Geometry: final body of the model. Coordinates: model frame, mm. Face numbers are marked on the shaded views. A direction names the side the tool comes from. Give positions to 0.01 mm unless a question says otherwise; leave off trailing zeros. Write each loop counter-clockwise with the first axis right and the second up, starting at its lowest first coordinate (ties: lowest second). Pieces come first, ordered by that corner, then holes.
Q1. Section B-B (x = -79). Return the cut outline in (y, z), plus the area to 3 significant figures.
Q2. Line query: line 1 (Y direction, x = -1.5, z = 42); line 2 (Z direction, x = -93, y = -549.5); line 3 (X direction, y = -310, z = 15). Output: solid intervals per line, ascending.
Q3. Section C-C (y = -154.5). Return the cut outline in (x, z), plus the area to 3 significant figures.
Q4. Section D-D (y = -1123.5). Return the cut outline in (x, z), plus the area to 3 significant figures.
Q5. Section A-A (z = 42). Return the cut outline in (x, y).
Q6. Pin query (flat end, axial travel): pin 1 Ø20.5 at (y, z) = (-846.67, 42) entering from -X; pin 2 Ø3 at (y, z) = (-1386.5, 1.5) entering from -X; pin 3 Ø1.5 at (y, z) = (-871, 23.5) entering from +X; pin 4 Ø16 at (y, z) = (-350, 42) entering from +X. Return the tip coordinate at first contact, or that it passes through.
Q7. Reachability of the marked faces 1 and 2 from +Z, -Z, +X, -X, +Y, -Y: full face, straight path, thin tool, end or side. Return the list, or none.
Autodesk Inventor part; units mm, degrees
ref_plane "YZ Plane" through (0, 0, 0) normal (1, 0, 0) x (0, 1, 0)
ref_plane "XZ Plane" through (0, 0, 0) normal (0, 1, 0) x (-1, 0, 0)
ref_plane "XY Plane" through (0, 0, 0) normal (0, 0, 1) x (1, 0, 0)
sketch "Sketch1" plane through (0, 0, 0) normal (0, 0, 1) x (1, 0, 0)
  line L0 (0, 0) -> (-122.6558, 0)
  line L1 (-122.6558, 0) -> (-122.6558, -1489.5)
  line L2 (-122.6558, -1489.5) -> (0, -1489.5)
  line L3 (0, -1489.5) -> (0, 0)
  line L4 (-122.6558, -1389.5) -> (-66, -1389.5)
  line L5 (-66, -1389.5) -> (-66, -1384.5)
  line L6 (-66, -1384.5) -> (-122.6558, -1384.5)
  line L7 (-122.6558, -1384.5) -> (-122.6558, -1389.5)
  line L8 (-122.6558, -893) -> (-66, -893)
  line L9 (-66, -893) -> (-66, -888)
  line L10 (-66, -888) -> (-122.6558, -888)
  line L11 (-122.6558, -888) -> (-122.6558, -893)
  line L12 (-122.6558, -396.5) -> (-66, -396.5)
  line L13 (-66, -396.5) -> (-66, -391.5)
  line L14 (-66, -391.5) -> (-122.6558, -391.5)
  line L15 (-122.6558, -391.5) -> (-122.6558, -396.5)
  circle A0 centre (-122.6558, -154.5) radius 30
  point P0 (-122.6558, -391.5)
  point P1 (-122.6558, -124.5)
  point P2 (-122.6558, -184.5)
  dimension "d0" = 1489.5
  dimension "d1" = 122.6559
  dimension "d2" = 5
  dimension "d4" = 100
  dimension "d7" = 496.5
  dimension "d23" = 66
  dimension "d28" = 60
  dimension "d29" = 1335
extrude "Plate1" add sketch "Sketch1" along normal blind 4 contours L3 L2 L1 L4 L5 L6 L8 L9 L10 L12 L13 L14 A0 L0
sketch "Sketch2" plane through (-4, 0, 0) normal (1, 0, 0) x (0, 1, 0)
  line L0 (-1489.5, 0) -> (0, 0)
  line L1 (0, 0) -> (0, 60)
  line L2 (0, 60) -> (-1489.5, 60)
  line L3 (-1489.5, 60) -> (-1489.5, 0)
edge flange "Flange1" height 60 angle 90 thickness 4 bend radius 4 thickness toward (1, 0, 0) relief tear relief width 4 relief depth 2 edges at (0, -744.75, 4) wall of the first edge with corners at (-4, -1489.5, 0) (-4, 0, 0) (-4, 0, 60) (-4, -1489.5, 60)
bend "Bend1"
corner "Corner1"
chamfer "Corner Chamfer1" distance 3 angle 45 6 edges at (-122.6558, -1389.5, 2) (-122.6558, -1384.5, 2) (-122.6558, -893, 2) (-122.6558, -888, 2) (-122.6558, -391.5, 2) (-122.6558, -396.5, 2)
sketch "Sketch4" plane through (0, -1489.5, 60) normal (1, 0, 0) x (0, 0, -1)
  circle A0 centre (18, 1139.5) radius 9
  line L0 (0, 0) -> (0, 1489.5)
  circle A1 centre (18, 642.8333) radius 9
  circle A2 centre (18, 146.1667) radius 9
  point P0 (60, 1489.5)
  dimension "d30" = 18
  dimension "d31" = 18
  dimension "d32" = 350
  dimension "d35" = 496.6667
extrude "Cut1" cut sketch "Sketch4" against normal blind 4
equation "\"d0\" = Стрингер_длина"
equation "\"d1\" = стрингер_глубина_7"
equation "\"d2\" = паз_под_стрингер_толщина"
equation "\"d7\" = 0.333333 * Стрингер_длина"
equation "\"d23\" = паз_под_стрингер_глубина - Thickness"
equation "\"d28\" = 2 * радиус_выреза_под_сварку"
equation "\"d35\" = Шаг_шпангоутов"
equation "\"d40\" = Thickness"
equation "\"d12\" = Thickness"
equation "\"d13\" = BendReliefWidth"
equation "\"d14\" = BendReliefDepth"
equation "\"d15\" = MinimumRemnant"
equation "\"d16\" = TransitionRadius"
equation "\"d17\" = ребро_усилителей"
equation "\"d19\" = BendRadius"
equation "\"d20\" = CornerReliefSize"
equation "\"d21\" = GapSize"
equation "\"d22\" = JacobiRadiusSize"
equation "\"BendRadius\" = Thickness"
equation "\"BendReliefWidth\" = Thickness"
equation "\"BendReliefDepth\" = 0.5 * Thickness"
equation "\"CornerReliefSize\" = 4 * Thickness"
equation "\"MinimumRemnant\" = 2 * Thickness"
equation "\"TransitionRadius\" = BendRadius"
equation "\"JacobiRadiusSize\" = BendRadius"
equation "\"GapSize\" = Thickness"
properties part number "GBK 0302 stringer 7" material "Steel"
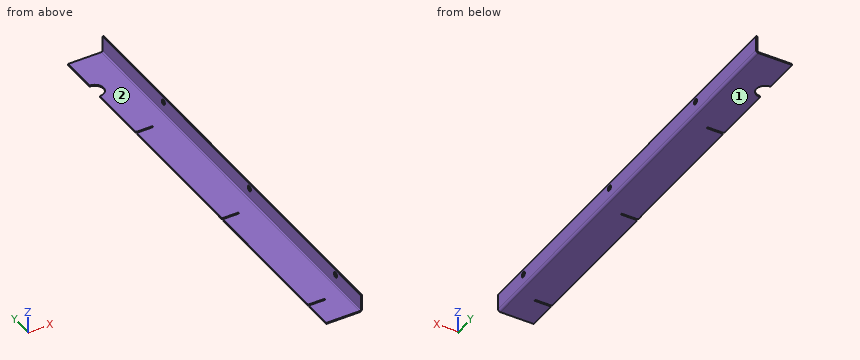
Computed:
1. outline: (-1489.5, 0) - (-1389.5, 0) - (-1389.5, 4) - (-1489.5, 4) - close; (-1384.5, 0) - (-893, 0) - (-893, 4) - (-1384.5, 4) - close; (-888, 0) - (-396.5, 0) - (-396.5, 4) - (-888, 4) - close; (-391.5, 0) - (0, 0) - (0, 4) - (-391.5, 4) - close
1. area: 5,900 mm2
2. line 1: y = -1489.5 to -1352.33, -1334.33 to -855.67, -837.67 to -359, -341 to 0
2. line 2: z = 0 to 4
2. line 3: x = -4 to 0
3. outline: (-92.66, 0) - (-8, 0) arc R8 ccw to (0, 8) - (0, 60) - (-4, 60) - (-4, 8) arc R4 cw to (-8, 4) - (-92.66, 4) - close
3. area: 584 mm2
4. outline: (-122.66, 0) - (-8, 0) arc R8 ccw to (0, 8) - (0, 60) - (-4, 60) - (-4, 8) arc R4 cw to (-8, 4) - (-122.66, 4) - close
4. area: 704 mm2
5. outline: (-4, -1489.5) - (0, -1489.5) - (0, -1352.33) - (-4, -1352.33) - close; (-4, -1334.33) - (0, -1334.33) - (0, -855.67) - (-4, -855.67) - close; (-4, -837.67) - (0, -837.67) - (0, -359) - (-4, -359) - close; (-4, -341) - (0, -341) - (0, 0) - (-4, 0) - close
6. pin 1: stops at x = -4
6. pin 2: stops at x = -66
6. pin 3: stops at x = 0
6. pin 4: passes through
7. face 1: -Z, +X, -X, +Y, -Y
7. face 2: +Z, -X, +Y, -Y
